from build123d import *

# Parameters (mm, degrees)
SKETCH_1_W                  = 323
SKETCH_1_H                  = 1746
SKETCH_1_R                  = 4.5
SKETCH_1_R_2                = 3.5
SKETCH_1_W_2                = 180
SKETCH_1_H_2                = 500
SM_BASE_FLANGE_1_DEPTH      = 2
SM_EDGE_FLANGE_1_DEPTH      = 1734
SM_EDGE_FLANGE_1_BEND_DEPTH = 1734
FILLET_1_R                  = 10
FILLET_2_R                  = 10


# Sheet-metal steps are written as plain solids
with BuildPart() as part:
    # Sketch 1 → Базовая кромка1 (new body)
    with BuildSketch(Plane(origin=(0, 0, 0), x_dir=(1, 0, 0), z_dir=(0, 1, 0))):
        Rectangle(SKETCH_1_W, SKETCH_1_H)
        with Locations(Location((-137.5, -765, 0), (0, 0, 270))):
            Circle(SKETCH_1_R, mode=Mode.SUBTRACT)
        with Locations(Location((137.5, -765, 0), (0, 0, 270))):
            Circle(SKETCH_1_R, mode=Mode.SUBTRACT)
        with Locations(Location((-137.5, -365, 0), (0, 0, 270))):
            Circle(SKETCH_1_R, mode=Mode.SUBTRACT)
        with Locations(Location((137.5, -365, 0), (0, 0, 270))):
            Circle(SKETCH_1_R, mode=Mode.SUBTRACT)
        with Locations(Location((-137.5, 35, 0), (0, 0, 270))):
            Circle(SKETCH_1_R, mode=Mode.SUBTRACT)
        with Locations(Location((137.5, 35, 0), (0, 0, 270))):
            Circle(SKETCH_1_R, mode=Mode.SUBTRACT)
        with Locations(Location((-137.5, 435, 0), (0, 0, 270))):
            Circle(SKETCH_1_R, mode=Mode.SUBTRACT)
        with Locations(Location((137.5, 435, 0), (0, 0, 270))):
            Circle(SKETCH_1_R, mode=Mode.SUBTRACT)
        with Locations(Location((-50, -527, 0), (0, 0, 270))):
            Circle(SKETCH_1_R_2, mode=Mode.SUBTRACT)
        with Locations(Location((50, -527, 0), (0, 0, 270))):
            Circle(SKETCH_1_R_2, mode=Mode.SUBTRACT)
        with Locations(Location((-50, 773, 0), (0, 0, 270))):
            Circle(SKETCH_1_R_2, mode=Mode.SUBTRACT)
        with Locations(Location((50, 773, 0), (0, 0, 270))):
            Circle(SKETCH_1_R_2, mode=Mode.SUBTRACT)
        with Locations((0, 123)):
            Rectangle(SKETCH_1_W_2, SKETCH_1_H_2, mode=Mode.SUBTRACT)
    extrude(amount=-SM_BASE_FLANGE_1_DEPTH)

    # Ребро-кромка1 section (across the edge) → Ребро-кромка1 (add)
    with BuildSketch(Plane(origin=(165.5, -2, -873), x_dir=(-1, 0, 0), z_dir=(0, 0, 1))):
        with BuildLine():
            Line((-2, 4), (-2, 38))
            Line((-2, 38), (0, 38))
            Line((0, 38), (0, 4))
            ThreePointArc((0, 4), (1.171572875, 1.171572875), (4, 0))
            Line((4, 0), (4, -2))
            ThreePointArc((4, -2), (-0.242640687, -0.242640687), (-2, 4))
        make_face()
    extrude(amount=SM_EDGE_FLANGE_1_DEPTH)

    # Ребро-кромка1 section 2 (across the edge) → Ребро-кромка1 bend (add)
    with BuildSketch(Plane(origin=(-165.5, -2, 861), x_dir=(1, 0, 0), z_dir=(0, 0, -1))):
        with BuildLine():
            Line((-2, 4), (-2, 38))
            Line((-2, 38), (0, 38))
            Line((0, 38), (0, 4))
            ThreePointArc((0, 4), (1.171572875, 1.171572875), (4, 0))
            Line((4, 0), (4, -2))
            ThreePointArc((4, -2), (-0.242640687, -0.242640687), (-2, 4))
        make_face()
    extrude(amount=SM_EDGE_FLANGE_1_BEND_DEPTH)

    # Скругление1
    fillet_1_edges = [part.edges().sort_by_distance(p)[0] for p in [
        (-166.5, -40, 861),
        (-166.5, -40, -873),
        (166.5, -40, -873),
        (166.5, -40, 861),
    ]]
    fillet(fillet_1_edges, radius=FILLET_1_R)

    # Скругление2
    fillet_2_edges = [part.edges().sort_by_distance(p)[0] for p in [
        (161.5, -1, 873),
        (-161.5, -1, 873),
    ]]
    fillet(fillet_2_edges, radius=FILLET_2_R)


solid = part.part
Work out the finished part from the listing and answer in its coordinate system (mm). A direction names the side the tool comes from. Round coordinates to 2 decimals unless told otherwise and drop trailing zeros. Loops run counter-clockwise (first coordinate to the right, second up) from the corner with the lowest first, then second, coordinate; pieces in that order, holes last. Notation, with made-up numbers: (3, 48) - (13, 48) arc R30 ccw to (13, 81) - close; hole circle Ø5 at (-19, 86). An arc over 180 degrees is marked (long way). One line per item, written item: value.
Q1. The mould has two halves that part along X. Classify faces 1 (the flat face through (167.5, -23, -18)), 2 (the flat face through (-167.5, -23, 6)), 3 (the flat face through (165.5, -23, -18)): +X half, -X half, draft (parallel to the pull), parting line (faces both ways), or undercut.
Check values:
face 1: +X half
face 2: -X half
face 3: undercut
Q2. Find section A-A on y = -17. Give the vertices of the cut face in (x, z), and give its area (3 significant figures).
Check values:
outline: (-167.5, -873) - (-165.5, -873) - (-165.5, 861) - (-167.5, 861) - close; (165.5, -873) - (167.5, -873) - (167.5, 861) - (165.5, 861) - close
area: 6,940 mm2
Q3. Straight lines are drawn through the part: probe 1 along X at (y, z) = (-1.4, 765); probe 2 along X at (y, z) = (-1.5, -35); probe 3 along Z at (x, y) = (-137, -1). For each, find the intervals that lie inside material, in ascending order.
Check values:
probe 1: -165.35 to -142, -133 to 133, 142 to 165.35
probe 2: -165.47 to -142, -133 to -90, 90 to 133, 142 to 165.47
probe 3: -873 to -439.47, -430.53 to -39.47, -30.53 to 360.53, 369.47 to 760.53, 769.47 to 873
Q4. Each of these flat-tipped pins is pushed along its axis until it touches: pin 1 Ø14.5 at (x, z) = (137.5, 765) entering from -Y; pin 2 Ø1 at (y, z) = (-1, 862) entering from +X; pin 3 Ø5 at (x, y) = (164, -15) entering from +Z. Where does it stop, or does it pass through?
Check values:
pin 1: y = -2
pin 2: x = 161.5
pin 3: z = 861
Q5. Find section B-B on z = -503. Give the vertices of the cut face in (x, y).
Check values:
outline: (-167.5, -40) - (-165.5, -40) - (-165.5, -6) arc R4 cw to (-161.5, -2) - (161.5, -2) arc R4 cw to (165.5, -6) - (165.5, -40) - (167.5, -40) - (167.5, -6) arc R6 ccw to (161.5, 0) - (-161.5, 0) arc R6 ccw to (-167.5, -6) - close
Q6. For faces 4 (the flat face through (-165.5, -23, 6)), 5 (the flat face through (-110, 0, -12)), determine the directions among +Z, -Z, +X, -X, +Y, -Y from which every point of the face is accessible in a straight line to the end or side of a thin tool.
Check values:
face 4: +Z, -Z, -Y
face 5: +Z, -Z, +X, -X, +Y
